Check sheet for the drawn part. Datum: minimum x, y, z corner. Units: mm. A direction names the side the tool comes from. Coordinates: 2 decimals unless noted, no trailing zeros. Order: outer loops, then holes, each group sorted by start corner. A loop starts at its lowest first (then second) coordinate and runs counter-clockwise, first axis right, second up. Notation, with made-up numbers: M -27,-14 L 30,-14 A32 cw 30,16 Z; hole C -19,7 d7. An arc over 180 degrees is marked long. Answer in a Markdown table with one row per item. Add a question column.
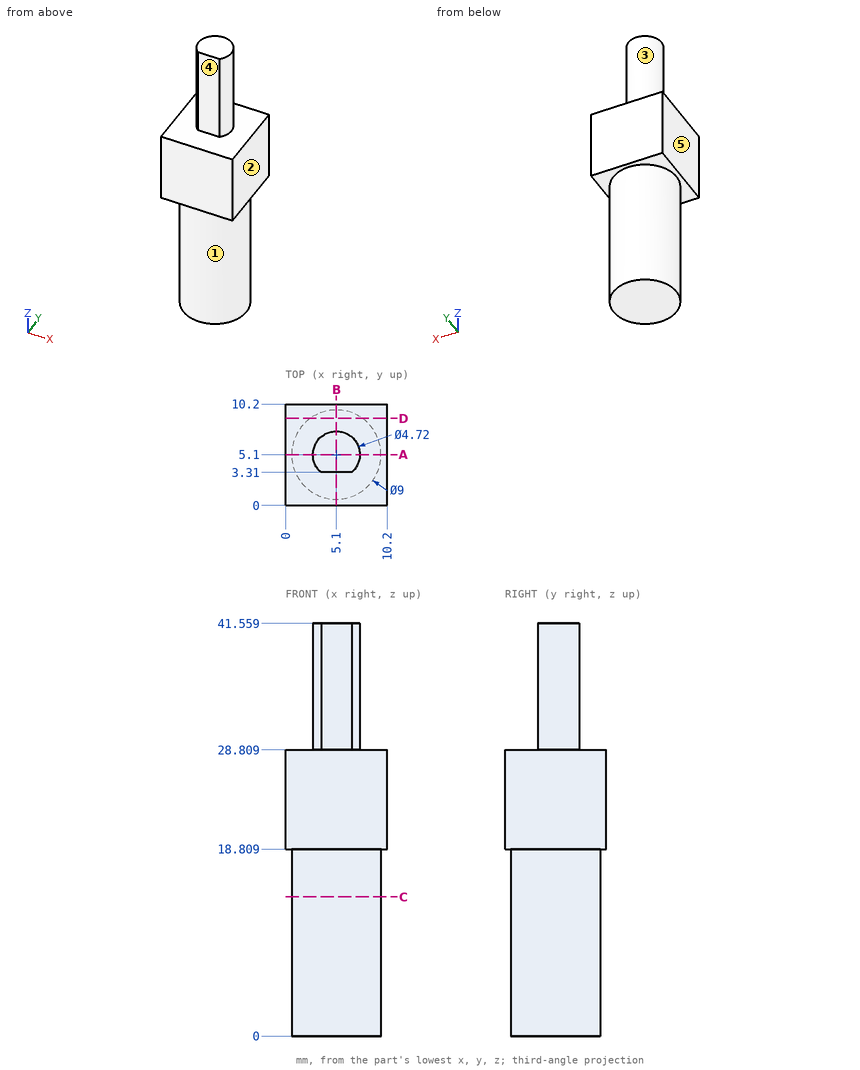
1. Section check D-D on y = 8.75. Enter the section's corners in (x, z).
2. Go/stop test with flat-tipped pins: pin 1 Ø0.9 at (x, z) = (5.5, 32) entering from -Y; pin 2 Ø2 at (x, z) = (2, 30) entering from -Y (1 decimal); pin 3 Ø1 at (y, z) = (7, 13.5) entering from +X; pin 4 Ø1 at (x, z) = (2, 32.5) entering from +Y. Record where each tip stops, or that it passes through.
3. Set-up check for the marked faces 1, 2, 3, 4 and 5: record each of +Z, -Z, +X, -X, +Y, -Y from which the full face is reachable in a straight line by a thin tool's end or side.
4. Section check B-B on x = 5.1. Enter the section's corners in (y, z).
5. Scan lines: line 1 (Z direction, x = 3, y = 6.25); line 2 (Z direction, x = 2.25, y = 1.25); line 3 (X direction, y = 5.25, z = 6). Record each from-to range of solid material in increasing order.
6. Section check C-C on z = 14. Enter the section's corners in (x, y), then the cut area to 3 significant figures.
7. Section check A-A on y = 5.1. Enter the section's corners in (x, z).
Result sheet:
| question | item | result |
|---|---|---|
| 1 | outline | M 0,18.81 L 2.47,18.81 L 2.47,0 L 7.73,0 L 7.73,18.81 L 10.2,18.81 L 10.2,28.81 L 0,28.81 Z |
| 2 | pin 1 | y = 3.31 |
| 2 | pin 2 | y = 4 |
| 2 | pin 3 | x = 9.38 |
| 2 | pin 4 | through |
| 3 | face 1 | -Z |
| 3 | face 2 | +Z, -Z, +X, +Y, -Y |
| 3 | face 3 | +Z |
| 3 | face 4 | +Z, +X, -X, -Y |
| 3 | face 5 | +Z, -Z, -X, +Y, -Y |
| 4 | outline | M 0,18.81 L 0.6,18.81 L 0.6,0 L 9.6,0 L 9.6,18.81 L 10.2,18.81 L 10.2,28.81 L 7.46,28.81 L 7.46,41.56 L 3.31,41.56 L 3.31,28.81 L 0,28.81 Z |
| 5 | line 1 | 0 to 28.81 |
| 5 | line 2 | 18.81 to 28.81 |
| 5 | line 3 | 0.6 to 9.6 |
| 6 | outline | C 5.1,5.1 d9 |
| 6 | area | 63.6 mm^2 |
| 7 | outline | M 0,18.81 L 0.6,18.81 L 0.6,0 L 9.6,0 L 9.6,18.81 L 10.2,18.81 L 10.2,28.81 L 7.46,28.81 L 7.46,41.56 L 2.74,41.56 L 2.74,28.81 L 0,28.81 Z |
